The listing builds one solid part. Answer for the finished solid, in the listing's coordinates (mm). A direction names the side the tool comes from. Coordinates: 2 decimals unless noted, no trailing zeros. Order: outer loops, then holes, each group sorted by start corner. A loop starts at its lowest first (then second) coordinate and runs counter-clockwise, first axis right, second up. Notation, with made-up numbers: M 37,53.25 L 92,53.25 A22 ccw 92,66.25 Z; hole C -21,-31.75 d9. An arc over 180 degrees is marked long. One line per item, written item: value. Start each with the question number.
Q1. Each of these flat-tipped pins is pushed along its axis until it touches: pin 1 Ø1.1 at (x, y) = (3.5, -2.5) entering from -Z; pin 2 Ø1.8 at (x, y) = (-4, 6) entering from -Z. Where does it stop, or does it pass through?
Q2. For faces 1 (the flat face through (-14.5, 2, 3)), 2 (the flat face through (-16, 2, 4)), 3 (the cylindrical face through (3.028, 3.006, 8.986)), determine the directions among +Z, -Z, +X, -X, +Y, -Y from which every point of the face is accessible in a straight line to the end or side of a thin tool.
Q3. The part is cut by section A-A on z = 5.25. Give the vertices of the cut face in (x, y).
Q4. The part is cut by section C-C on y = 2.5. Give the vertices of the cut face in (x, z), then the cut area to 3 significant figures.
Q5. Determine the mould class of faces 4 (the cylindrical face through (13.975, -1.299, 8.986)), 5 (the flat face through (0, -6.374, 4)), 6 (the flat face through (-12, 6, 10)) for opening direction Y: pulls with the +Y half, pulls with the -Y half, needs draft (parallel to the pull), parting line crosses it, or undercut.
Q6. The part is cut by section D-D on z = 7. Give the number of separate pieces and of enclosed holes in the cut face, then the cut area to 3 significant figures.
Q7. The part is cut by section B-B on x = -8. Give the vertices of the cut face in (y, z).
Q8. Straight lines are drawn through the part: line 1 along Y through (x, z) = (-12.5, 6.75); line 2 along X through (y, z) = (5.5, 7); line 3 along X through (y, z) = (4.5, 1.75). For each, find the intervals that lie inside material, in ascending order. Write a range as [from, to].
```python
from build123d import *

# Parameters (mm, degrees)
F0_W     = 32
F0_H     = 16
F1_DEPTH = 8
F3_R     = 2.5890653677
F3_R_2   = 2.5126878493
F3_R_3   = 2.6441660213
F3_R_4   = 2.5038047819
F3_R_5   = 2.6210090881
F3_R_6   = 2.500461059
F3_R_7   = 2.6359235988
F3_R_8   = 2.5954418061
F4_DEPTH = 2
F5_R     = 0.5
F6_R     = 0.5
F7_R     = 0.5
F8_T     = -1.5


with BuildPart() as f1:
    # F0 (on Top) → F1 (new body)
    with BuildSketch(Plane.XY):
        with Locations((0, 1.6263736921)):
            Rectangle(F0_W, F0_H)
    extrude(amount=F1_DEPTH)

    # F3 (on offset) → F4 (join)
    with BuildSketch(Plane.XY.offset(8)):
        with Locations((3.5897120633, 5.5338214714)):
            Circle(F3_R)
        with Locations((-12.4102879367, 5.5338214714)):
            Circle(F3_R_2)
        with Locations((-4.4102879367, 5.5338214714)):
            Circle(F3_R_3)
        with Locations((-12.4102879367, -2.0500652119)):
            Circle(F3_R_4)
        with Locations((11.5897120633, 5.5338214714)):
            Circle(F3_R_5)
        with Locations((11.5897120633, -2.0500652119)):
            Circle(F3_R_6)
        with Locations((3.5897120633, -2.0500652119)):
            Circle(F3_R_7)
        with Locations((-4.4102879367, -2.0500652119)):
            Circle(F3_R_8)
    extrude(amount=F4_DEPTH)

    # F5
    f5_edges = [f1.edges().sort_by_distance(p)[0] for p in [
        (-16, 9.626374, 4),
    ]]
    fillet(f5_edges, radius=F5_R)

    # F6
    f6_edges = [f1.edges().sort_by_distance(p)[0] for p in [
        (16, 9.626374, 4),
    ]]
    fillet(f6_edges, radius=F6_R)

    # F7
    f7_edges = [f1.edges().sort_by_distance(p)[0] for p in [
        (16, -6.373626, 4),
        (-16, -6.373626, 4),
    ]]
    fillet(f7_edges, radius=F7_R)

    # F8
    f8_openings = [f1.faces().sort_by_distance(p)[0] for p in [
        (0, 1.626374, 0),
    ]]
    offset(amount=F8_T, openings=f8_openings, kind=Kind.INTERSECTION)


solid = f1.part
```
Output:
1. pin 1: stops at z = 8.5
1. pin 2: stops at z = 6.5
2. face 1: -Z
2. face 2: +Z, -Z, -X, +Y, -Y
2. face 3: +Z
3. outline: M -16,-5.87 A0.5 ccw -15.5,-6.37 L 15.5,-6.37 A0.5 ccw 16,-5.87 L 16,9.13 A0.5 ccw 15.5,9.63 L -15.5,9.63 A0.5 ccw -16,9.13 Z; hole M -14.5,-4.87 L 14.5,-4.87 L 14.5,8.13 L -14.5,8.13 Z
4. outline: M -16,0 L -14.5,0 L -14.5,6.5 L 14.5,6.5 L 14.5,0 L 16,0 L 16,8 L -16,8 Z
4. area: 67.5 mm^2
5. face 4: undercut
5. face 5: pulls with the -Y half
5. face 6: needs draft
6. separate pieces: 1
6. enclosed holes: 8
6. area: 483 mm^2
7. outline: M -6.37,0 L -4.87,0 L -4.87,6.5 L 8.13,6.5 L 8.13,0 L 9.63,0 L 9.63,8 L -6.37,8 Z
8. line 1: y = [-6.37, -3.05], [-1.05, 4.53], [6.54, 9.63]
8. line 2: x = [-16, -13.42], [-11.4, -5.55], [-3.27, 2.5], [4.68, 10.47], [12.71, 16]
8. line 3: x = [-16, -14.5], [14.5, 16]
